Autodesk Inventor part; units mm, degrees
ref_plane "YZ Plane" through (0, 0, 0) normal (1, 0, 0) x (0, 1, 0)
ref_plane "XZ Plane" through (0, 0, 0) normal (0, 1, 0) x (-1, 0, 0)
ref_plane "XY Plane" through (0, 0, 0) normal (0, 0, 1) x (1, 0, 0)
sketch "Sketch1" plane through (0, 0, 0) normal (0, 1, 0) x (-1, 0, 0)
  line L0 (-28.2, -28.2) -> (28.2, -28.2)
  line L1 (28.2, -28.2) -> (28.2, 28.2)
  line L2 (28.2, 28.2) -> (-28.2, 28.2)
  line L3 (-28.2, 28.2) -> (-28.2, -28.2)
  line L4 (-28.2, -28.2) -> (28.2, 28.2) construction
  line L5 (28.2, -28.2) -> (-28.2, 28.2) construction
  line L6 (-23.55, 23.55) -> (23.55, 23.55) construction
  line L7 (23.55, 23.55) -> (23.55, -23.55) construction
  line L8 (23.55, -23.55) -> (-23.55, -23.55) construction
  line L9 (-23.55, -23.55) -> (-23.55, 23.55) construction
  line L10 (-23.55, 23.55) -> (23.55, -23.55) construction
  line L11 (23.55, 23.55) -> (-23.55, -23.55) construction
  circle A0 centre (23.55, 23.55) radius 2
  circle A1 centre (23.55, -23.55) radius 2
  circle A2 centre (-23.55, -23.55) radius 2
  circle A3 centre (-23.55, 23.55) radius 2
  circle A4 centre (0, 0) radius 20
  line L12 (28.2, 28.2) -> (-28.2, 28.2)
  line L13 (-28.2, 28.2) -> (-28.2, 38.2)
  line L14 (-28.2, 38.2) -> (28.2, 38.2)
  line L15 (28.2, 38.2) -> (28.2, 28.2)
  dimension "d0" = 56.4
  dimension "d1" = 56.4
  dimension "d2" = 47.1
  dimension "d3" = 47.1
  dimension "d4" = 4
  dimension "d5" = 4
  dimension "d6" = 4
  dimension "d7" = 4
  dimension "d8" = 40
  dimension "d16" = 10
extrude "Extrusion1" add sketch "Sketch1" along normal blind 24 contours L3 L2 L1 L0
sketch "Sketch2" plane through (0, 24, 0) normal (0, 1, 0) x (1, 0, 0)
  circle A0 centre (0, 0) radius 20
  circle A1 centre (23.55, -23.55) radius 2
  circle A2 centre (23.55, 23.55) radius 2
  circle A3 centre (-23.55, 23.55) radius 2
  circle A4 centre (-23.55, -23.55) radius 2
  line L0 (28.2, 28.2) -> (-28.2, 28.2)
  line L1 (-28.2, 28.2) -> (-28.2, -28.2)
  line L2 (28.2, -28.2) -> (28.2, 28.2)
  circle A5 centre (0, 0) radius 6.5
  line L3 (-6.4978, 0.1686) -> (-26.2939, -54.2207)
  line L4 (-6.4978, 0.1686) -> (51.3822, 0.1686) construction
  line L5 (6.4521, -0.788) -> (25.9, -54.2207)
  line L6 (6.4521, -0.788) -> (63.314, -0.788) construction
  line L7 (25.9, -54.2207) -> (-26.2939, -54.2207)
  line L8 (-28.2, -28.2) -> (28.2, -28.2)
  dimension "d11" = 110
  dimension "d12" = 70
  dimension "d13" = 13
extrude "Extrusion2" cut sketch "Sketch2" against normal blind 15 contours L3 A5 L5 A0 | A0 L5 L8 L3 | A5 | L8 L5 L7 L3 picked at (-8.2958, -12.9873)
sketch "Sketch3" plane through (-28.2, 0, -28.2) normal (-1, 0, 0) x (0, 0, 1)
  line L0 (0, 0) -> (56.4, 0)
  line L1 (0, 24) -> (56.4, 24)
  line L2 (0, 0) -> (0, 24)
  line L3 (49.75, 24) -> (53.75, 24)
  line L4 (53.75, 0) -> (49.75, 0)
  line L5 (2.65, 24) -> (6.65, 24)
  line L6 (6.65, 0) -> (2.65, 0)
  line L7 (6.65, 0) -> (6.65, 24)
  line L8 (2.65, 0) -> (2.65, 24)
  line L9 (49.75, 0) -> (49.75, 24)
  line L10 (53.75, 0) -> (53.75, 24)
  line L11 (56.4, 0) -> (56.4, 24)
  point P0 (28.2, 0)
sketch "Sketch4" plane through (-28.2, 0, -28.2) normal (-1, 0, 0) x (0, 0, 1)
  line L0 (0, 0) -> (56.4, 0)
  line L1 (0, 24) -> (56.4, 24)
  line L2 (0, 0) -> (0, 24)
  circle A0 centre (4, 14) radius 2.5
  circle A1 centre (46, 14) radius 2.5
  line L3 (4.5098, 0) -> (4.5098, 24) construction
  line L4 (0, 24) -> (66.4, 24) construction
  line L5 (56.4, 0) -> (56.4, 24)
  point P0 (28.2, 0)
  dimension "d17" = 5
  dimension "d18" = 5
  dimension "d19" = 4.5098
  dimension "d20" = 4
  dimension "d21" = 14
  dimension "d22" = 0
  dimension "d23" = 42
hole "Hole1" at (-28.2, 14, -24.2) at (-28.2, 14, 17.8) direction (1, 0, 0) diameter 4 depth 16 tip angle 118
sketch "Sketch5" plane through (0, 24, 0) normal (0, 1, 0) x (1, 0, 0)
  line L0 (-16.8232, -28.2) -> (-12.2994, -15.771)
  arc A0 (11.9912, -16.0066) -> (-12.2994, -15.771) centre (0, 0) ccw
  line L1 (11.9912, -16.0066) -> (16.4292, -28.2)
  line L2 (28.2, -28.2) -> (28.2, 28.2)
  line L3 (28.2, 28.2) -> (-28.2, 28.2)
  line L4 (-28.2, 28.2) -> (-28.2, -28.2)
  circle A1 centre (23.55, -23.55) radius 2
  circle A2 centre (23.55, 23.55) radius 2
  circle A3 centre (-23.55, 23.55) radius 2
  circle A4 centre (-23.55, -23.55) radius 2
  line L5 (16.4292, -28.2) -> (28.2, -28.2)
  line L6 (-28.2, -28.2) -> (-16.8232, -28.2)
hole "Hole2" at (-23.55, 24, 23.55) at (-23.55, 24, -23.55) at (23.55, 24, -23.55) at (23.55, 24, 23.55) direction (0, -1, 0) diameter 4 depth 12 tip angle 118 counterbore diameter 8 counterbore depth 10
sketch "Sketch6" plane through (28.2, 0, -28.2) normal (0, 0, -1) x (-1, 0, 0)
  line L0 (41.2379, 16) -> (56.4, 16)
  line L1 (40.4, 12) -> (56.4, 12)
  line L2 (48.3294, 18.4358) -> (43.3294, 18.4358)
  line L3 (43.3294, 18.4358) -> (43.3294, 9.4358)
  line L4 (43.3294, 9.4358) -> (48.3294, 9.4358)
  line L5 (48.3294, 9.4358) -> (48.3294, 18.4358)
  line L6 (48.3294, 18.4358) -> (43.3294, 9.4358) construction
  line L7 (43.3294, 18.4358) -> (48.3294, 9.4358) construction
  point P0 (28.2, 0)
  point P1 (45.8294, 13.9358)
  dimension "d38" = 9
  dimension "d39" = 5
extrude "Extrusion3" cut sketch "Sketch6" against normal through all
properties part number "00_NEMA23_holder"
Read the model definition and answer for the solid it produces. Units are mm, in the model's axes. A direction names the side the tool comes from. Round coordinates to 2 decimals unless told otherwise and drop trailing zeros. Write each loop counter-clockwise with the first axis right and the second up, starting at its lowest first coordinate (ties: lowest second). Pieces come first, ordered by that corner, then holes.
1. The part is cut by section B-B, the plane z = 12. Determine the outline of the cut face in (x, y), then the cut area to 3 significant figures.
2. Determine the mould class of faces 1 (the face through (21.703, 6.902, 24.316)), 2 (the face through (-15.129, 14, 21)), 3 (the face through (19, 0, 7)) for opening direction Y: pulls with the +Y half, pulls with the -Y half, needs draft (parallel to the pull), parting line crosses it, or undercut.
3. The part is cut by section C-C, the plane x = 23.55. Determine the outline of the cut face in (y, z).
4. The part is cut by section D-D, the plane x = 0. Determine the outline of the cut face in (y, z).
5. The part is cut by section A-A, the plane y = 11. Determine the outline of the cut face in (x, z), then the cut area to 3 significant figures.
6. Which of the six approach directions +Z, -Z, +X, -X, +Y, -Y give full straight-line access (tool end or side, diameter ignored) to faces 4 (the face through (13, 24, -18)), 5 (the face through (-19, 18.436, -7)), 6 (the face through (-25.005, 12.648, -25.674)), 7 (the face through (14.18, 16.6, 22.02)), 8 (the face through (20.85, 18.93, -26.5))?
7. Given pin 1 Ø2.5 at (x, z) = (24, 22) entering from +Y; pin 2 Ø3 at (y, z) = (14, -24.2) entering from -X; pin 3 Ø3.5 at (y, z) = (14, 17.8) entering from -X, each flat-ended and moving along its own axis, determine where each tip first touches the part or whether it passes through.
8. Straight lines are drawn through the part: L1, parallel to Z at x = -23.55, y = 4.25; L2, parallel to X at y = 18, z = -23.55; L3, parallel to X at y = 17, z = -18. For each, find the intervals that lie inside material, in ascending order.
Values:
1. outline: (-28.2, 0) - (-16, 0) - (-16, 9.44) - (-20.13, 9.44) - (-20.13, 18.44) - (-16, 18.44) - (-16, 24) - (-28.2, 24) - close; (16, 0) - (28.2, 0) - (28.2, 24) - (16, 24) - close
1. area: 548 mm2
2. face 1: needs draft
2. face 2: undercut
2. face 3: pulls with the -Y half
3. outline: (0, -28.2) - (24, -28.2) - (24, -27.55) - (14, -27.55) - (14, -25.55) - (0, -25.55) - close; (0, -21.55) - (14, -21.55) - (14, -19.55) - (24, -19.55) - (24, 19.55) - (14, 19.55) - (14, 21.55) - (0, 21.55) - close; (0, 25.55) - (14, 25.55) - (14, 27.55) - (24, 27.55) - (24, 28.2) - (0, 28.2) - close
4. outline: (0, -28.2) - (24, -28.2) - (24, -20) - (0, -20) - close; (0, 20) - (9, 20) - (9, 28.2) - (0, 28.2) - close
5. outline: (-28.2, -28.2) - (-20.13, -28.2) - (-20.13, 28.2) - (-28.2, 28.2) - close; (-15.13, -28.2) - (28.2, -28.2) - (28.2, 28.2) - (16.43, 28.2) - (11.99, 16.01) arc R20 cw (long way) to (-15.13, -13.08) - close; (-15.13, 13.08) arc R20 cw to (-12.3, 15.77) - (-15.13, 23.55) - close; hole circle Ø4 at (-23.55, -23.55); hole circle Ø4 at (-23.55, 23.55); hole circle Ø4 at (23.55, -23.55); hole circle Ø4 at (23.55, 23.55)
5. area: 1,400 mm2
6. face 4: +Z, -Z, +X, -X, +Y
6. face 5: +Z, -Z
6. face 6: -X
6. face 7: +Z, +Y
6. face 8: +Y
7. pin 1: stops at y = 14
7. pin 2: stops at x = -11.9
7. pin 3: stops at x = 12.01
8. L1: z = -28.2 to -25.55, -21.55 to 21.55, 25.55 to 28.2
8. L2: x = -28.2 to -27.55, -15.13 to 19.55, 27.55 to 28.2
8. L3: x = -28.2 to -20.13, -15.13 to -8.72, 8.72 to 28.2
